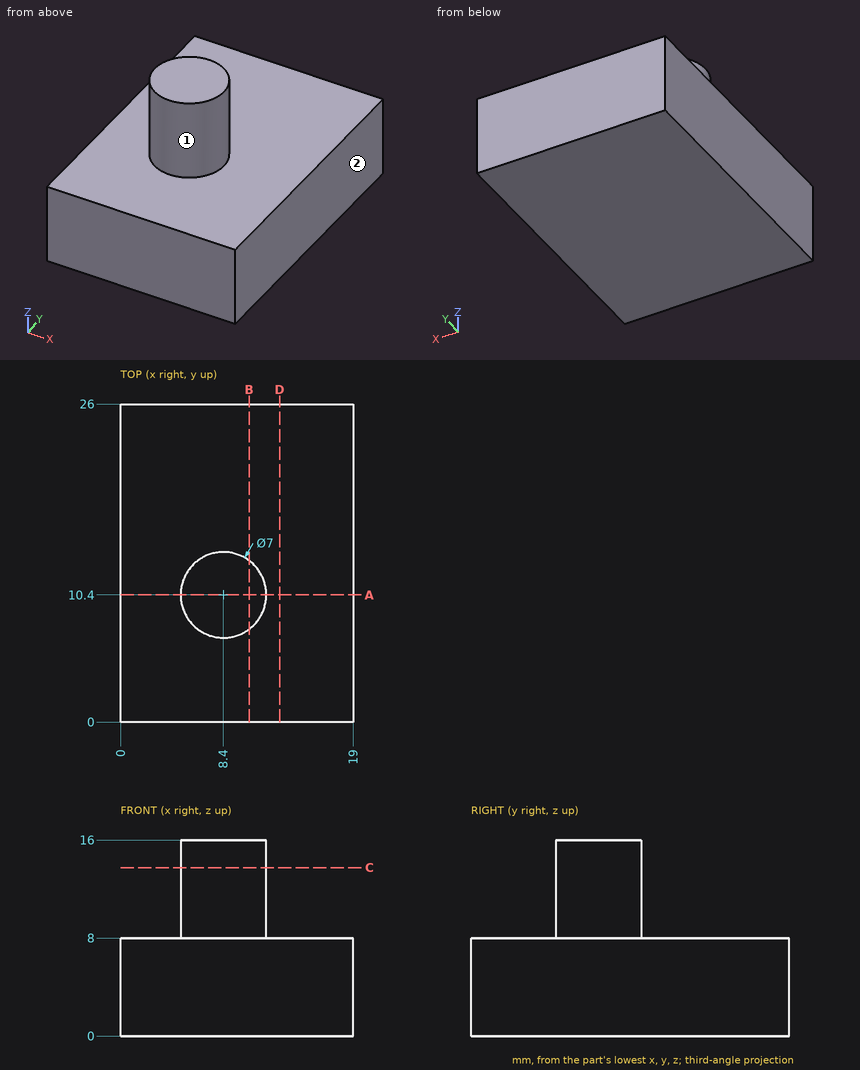
Study the drawing (mm; zero at the part's minimum x, y, z) and answer. A direction names the side the tool comes from. Round coordinates to 2 decimals unless told otherwise and drop trailing zeros. Write each loop counter-clockwise with the first axis right and the second up, starting at its lowest first coordinate (ties: lowest second). Pieces come first, ordered by that corner, then holes. Notation, with made-up numbers: (59, 69.5) - (77, 69.5) arc R23 ccw to (77, 96.5) - close; hole circle Ø5 at (11.5, -5). An arc over 180 degrees is marked (long way). Use CSV: the item, a comma, the result in double quotes.
Q1. A tool of negligible diameter and unlimited length cuts with its end or side. For the marked faces 1 and 2, from which of +Z, -Z, +X, -X, +Y, -Y can it reach the whole face along a straight path? Write none if from no direction.
Values:
face 1,"+Z"
face 2,"+Z, -Z, +X, +Y, -Y"
Q2. Find section A-A, the plane y = 10.4. Write down the section's boundary in (x, z).
Values:
outline,"(0, 0) - (19, 0) - (19, 8) - (11.9, 8) - (11.9, 16) - (4.9, 16) - (4.9, 8) - (0, 8) - close"
Q3. Straight lines are drawn through the part: line 1 along Z through (x, y) = (13.5, 14); line 2 along X through (y, z) = (10.5, 15.25); line 3 along X through (y, z) = (11.5, 13). For each, find the intervals that lie inside material, in ascending order.
Values:
line 1,"z = 0 to 8"
line 2,"x = 4.9 to 11.9"
line 3,"x = 5.08 to 11.72"
Q4. Find section D-D, the plane x = 13. Write down the section's boundary in (y, z), then the cut area to 3 significant figures.
Values:
outline,"(0, 0) - (26, 0) - (26, 8) - (0, 8) - close"
area,"208 mm²"
Q5. Find section B-B, the plane x = 10.5. Write down the section's boundary in (y, z).
Values:
outline,"(0, 0) - (26, 0) - (26, 8) - (13.2, 8) - (13.2, 16) - (7.6, 16) - (7.6, 8) - (0, 8) - close"
Q6. Find section C-C, the plane z = 13.75. Write down the section's boundary in (x, y), then the cut area to 3 significant figures.
Values:
outline,"circle Ø7 at (8.4, 10.4)"
area,"38.5 mm²"
Q7. Each of these flat-tipped pins is pushed along its axis until it touches: pin 1 Ø5 at (y, z) = (16, 13) entering from -X; pin 2 Ø2 at (y, z) = (4, 12) entering from +X; pin 3 Ø1 at (x, y) = (5.5, 17.5) entering from +Z. Where does it stop, or does it pass through?
Values:
pin 1,"stops at x = 6.78"
pin 2,"passes through"
pin 3,"stops at z = 8"
